from build123d import *

# Parameters (mm, degrees)
SKETCH1_W               = 85
SKETCH1_H               = 85
SKETCH1_W_2             = 20
SKETCH1_H_2             = 25
BOSS_EXTRUDE1_DEPTH     = 42
CUT_EXTRUDE1_DEPTH      = 108.686284851
CUT_EXTRUDE2_DEPTH      = 122.642881801
CUT_EXTRUDE3_START      = -85
CUT_EXTRUDE3_DEPTH      = 85
SKETCH6_W               = 67
SKETCH6_H               = 42
CUT_EXTRUDE4_DEPTH      = 35
FILLET1_R               = 3
FILLET2_R               = 3
CUT_EXTRUDE6_DEPTH      = 107.514112815
CUT_EXTRUDE6_DEPTH_BACK = 107.514112815
M5_TAPPED_HOLE2_D       = 4.2
M5_TAPPED_HOLE2_DEPTH   = 8
M5_TAPPED_HOLE2_TIP     = 1.2618073
SKETCH17_R              = 2.5
CUT_EXTRUDE7_DEPTH      = 107.922102397


# Read off the part's stored shape, not the designer's step: Cut-Extrude3
with BuildPart() as part:
    # Sketch1 → Boss-Extrude1 (new body)
    with BuildSketch(Plane(origin=(0, 0, 0), x_dir=(1, 0, 0), z_dir=(0, 1, 0))):
        with Locations((-20.937727355, 33.710174471)):
            Rectangle(SKETCH1_W, SKETCH1_H)
        with Locations((-53.437727355, -21.289825529)):
            Rectangle(SKETCH1_W_2, SKETCH1_H_2)
        with Locations((11.562272645, -21.289825529)):
            Rectangle(SKETCH1_W_2, SKETCH1_H_2)
    extrude(amount=BOSS_EXTRUDE1_DEPTH)

    # Sketch2 → Cut-Extrude1 (cut, through all)
    with BuildSketch(Plane(origin=(0, 42, 0), x_dir=(1, 0, 0), z_dir=(0, 1, 0))):
        with BuildLine():
            Line((-63.437727355, -23.334516424), (-63.437727355, -33.789825529))
            Line((-63.437727355, -33.789825529), (-43.437727355, -33.789825529))
            Line((-43.437727355, -33.789825529), (-43.437727355, -23.334516424))
            ThreePointArc((-43.437727355, -23.334516424), (-53.437727355, -33.334516424), (-63.437727355, -23.334516424))
        make_face()
        with BuildLine():
            Line((1.562272645, -23.334516424), (1.562272645, -33.789825529))
            Line((1.562272645, -33.789825529), (21.562272645, -33.789825529))
            Line((21.562272645, -33.789825529), (21.562272645, -23.334516424))
            ThreePointArc((21.562272645, -23.334516424), (11.562272645, -33.334516424), (1.562272645, -23.334516424))
        make_face()
    extrude(amount=-CUT_EXTRUDE1_DEPTH, mode=Mode.SUBTRACT)

    # Sketch3 → Cut-Extrude2 (cut, through all)
    with BuildSketch(Plane.ZY.offset(63.437727355)):
        Polygon((33.334516424, 2), (15.334516424, 2), (10.589618013, 0), (33.334516424, 0), align=None)
        Polygon((15.334516424, 40), (10.589618013, 42), (33.334516424, 42), (33.334516424, 40), align=None)
    extrude(amount=-CUT_EXTRUDE2_DEPTH, mode=Mode.SUBTRACT)

    # Cut-Extrude3 outline → Cut-Extrude3 (cut)
    with BuildSketch(Plane.ZY.offset(63.437727355).offset(CUT_EXTRUDE3_START)):
        with BuildLine():
            Line((33.334516424, 5.260289026), (33.334516424, 36.739710974))
            Line((33.334516424, 36.739710974), (5.643342669, 36.739710974))
            ThreePointArc((5.643342669, 36.739710974), (-13.23093958, 21), (5.643342669, 5.260289026))
            Line((5.643342669, 5.260289026), (33.334516424, 5.260289026))
        make_face()
    extrude(amount=CUT_EXTRUDE3_DEPTH, mode=Mode.SUBTRACT)

    # Sketch6 → Cut-Extrude4 (cut)
    with BuildSketch(Plane(origin=(0, 0, -76.210174471), x_dir=(-1, 0, 0), z_dir=(0, 0, -1))):
        with Locations((20.937727355, 21)):
            Rectangle(SKETCH6_W, SKETCH6_H)
    extrude(amount=-CUT_EXTRUDE4_DEPTH, mode=Mode.SUBTRACT)

    # Fillet1
    # the kernel refuses this fillet: 3 mm, written as the material it takes off along each edge
    with BuildSketch(Plane(origin=(-63.437727355, 42, -94.210174471), x_dir=(1, 0, 0), z_dir=(0, 0, 1)), Plane(origin=(-63.437727355, 0, 28.589618013), x_dir=(1, 0, 0), z_dir=(0, 0, -1)), Plane(origin=(21.562272645, 42, -94.210174471), x_dir=(0, -1, 0), z_dir=(0, 0, 1)), Plane(origin=(21.562272645, 0, 28.589618013), x_dir=(0, 1, 0), z_dir=(0, 0, -1))) as fillet1_piece_1:
        with BuildLine():
            CenterArc((FILLET1_R, -FILLET1_R), FILLET1_R, 90, 90)
            Line((0, -FILLET1_R), (-FILLET1_R * 0.02, -FILLET1_R))
            Line((-FILLET1_R * 0.02, -FILLET1_R), (-FILLET1_R * 0.02, FILLET1_R * 0.02))
            Line((-FILLET1_R * 0.02, FILLET1_R * 0.02), (FILLET1_R, FILLET1_R * 0.02))
            Line((FILLET1_R, FILLET1_R * 0.02), (FILLET1_R, 0))
        make_face()
    extrude(amount=122.799792484, mode=Mode.SUBTRACT)

    # Fillet2
    fillet2_edges = [part.edges().sort_by_distance(p)[0] for p in [
        (12.562272645, 21, -41.210174471),
        (-54.437727355, 21, -41.210174471),
    ]]
    fillet(fillet2_edges, radius=FILLET2_R)

    # Sketch9 → Cut-Extrude6 (cut, two sides: drawn at the far end of the back side and taken through both)
    with BuildSketch(Plane(origin=(0, 0, -41.210174471), x_dir=(-1, 0, 0), z_dir=(0, 0, -1)).offset(-CUT_EXTRUDE6_DEPTH_BACK)):
        with BuildLine():
            Line((35.10328306, 7.804043613), (6.77217165, 7.804043613))
            ThreePointArc((6.77217165, 7.804043613), (3.236637744, 9.268509707), (1.77217165, 12.804043613))
            Line((1.77217165, 12.804043613), (1.77217165, 29.195956387))
            ThreePointArc((1.77217165, 29.195956387), (3.236637744, 32.731490293), (6.77217165, 34.195956387))
            Line((6.77217165, 34.195956387), (35.10328306, 34.195956387))
            ThreePointArc((35.10328306, 34.195956387), (38.638816966, 32.731490293), (40.10328306, 29.195956387))
            Line((40.10328306, 29.195956387), (40.10328306, 12.804043613))
            ThreePointArc((40.10328306, 12.804043613), (38.638816966, 9.268509707), (35.10328306, 7.804043613))
        make_face()
    extrude(amount=CUT_EXTRUDE6_DEPTH + CUT_EXTRUDE6_DEPTH_BACK, mode=Mode.SUBTRACT)

    # M5 Tapped Hole2
    with Locations(Plane(origin=(16.562272645, 29.5, -76.210174471), x_dir=(-1, 0, 0), z_dir=(0, 0, -1))):
        with Locations((0, 0), (0, -17), (75, -17), (75, 0)):
            Hole(M5_TAPPED_HOLE2_D / 2, depth=M5_TAPPED_HOLE2_DEPTH)
            with Locations((0, 0, -(M5_TAPPED_HOLE2_DEPTH + M5_TAPPED_HOLE2_TIP / 2))):  # 118° drill point
                Cone(0, M5_TAPPED_HOLE2_D / 2, M5_TAPPED_HOLE2_TIP, mode=Mode.SUBTRACT)

    # Sketch17 → Cut-Extrude7 (cut, through all)
    with BuildSketch(Plane(origin=(0, 40, 0), x_dir=(1, 0, 0), z_dir=(0, 1, 0))):
        with Locations(Location((-53.437727355, -24.203700837, 0), (0, 0, 270))):
            Circle(SKETCH17_R)
        with Locations(Location((11.562272645, -24.203700837, 0), (0, 0, 270))):
            Circle(SKETCH17_R)
    extrude(amount=-CUT_EXTRUDE7_DEPTH, mode=Mode.SUBTRACT)


solid = part.part
Could you check a few things on this model? Use its own coordinates, in mm. A direction names the side the tool comes from. Coordinates: 2 decimals unless noted, no trailing zeros. Order: outer loops, then holes, each group sorted by start corner. A loop starts at its lowest first (then second) coordinate and runs counter-clockwise, first axis right, second up. Notation, with made-up numbers: (-31.75, -21.5) - (5.25, -21.5) arc R7 cw to (5.25, -13.5) - close; hole circle Ø6 at (-35.75, 75.5). An arc over 180 degrees is marked (long way). Answer in a Markdown table with one row per item. Add a question column.
(1) If we section it at B-B, the plane y = 21: Please give me the cut outline in (x, z), then the cut area to 3 significant figures.
(2) If we section it at C-C, the plane x = -5.5: Please give me the cut outline in (y, z).
(3) I need wall thicknesses on L1, parallel to X at y = 29.5, z = -70; L2, parallel to X at y = 34, z = -65; L3, parallel to Y at x = -23.5, z = 7. Which ranges of each line are inside material? Lowest first, please.
(4) If we mould it in two halves opening along Y, with no side actions, what happens to faces 1 (the face through (1.562, 3, 16)), 2 (the face through (-21, 42, -24)), 3 (the face through (-38.68, 9.31, -23.5))? For each: released by +Y, released by -Y, zero draft, split by the parting line, or undercut.
(5) Will these pins go through, and if not, where does the flat tip stop? pin 1 (1 mm diameter, centred on x = -27.5, y = 8.5, fed in from +Z); pin 2 (5.5 mm diameter, centred on x = -58.44, y = 12.5, fed in from +Z); pin 3 (2.5 mm diameter, centred on y = 1.5, z = 13.5, fed in from -X); pin 4 (5.5 mm diameter, centred on x = 7.5, z = 26.5, fed in from -Y).
(6) If we section it at A-A, the plane z = -37.5: Please give me the cut outline in (x, y).
(7) If we section it at D-D, the plane z = 7.5: Please give me the cut outline in (x, y), then the cut area to 3 significant figures.
(8) On a 3-axis mill with a long thin cutter (end or side, diameter ignored), from which of +Z, -Z, +X, -X, +Y, -Y can I reach the whole of each face in a straight line? I mean faces 4 (the face through (12.562, 21, -60)), 5 (the face through (-20, 36.74, 7)), 6 (the face through (-38.6, 32.77, -23.5)), 7 (the face through (-56.498, 11.696, -72.154)), 8 (the face through (-43.438, 3, 16)). Say none if no direction works.
Results are:
| question | item | result |
|---|---|---|
| 1 | outline | (-63.44, -76.21) - (-54.44, -76.21) - (-54.44, -44.21) arc R3 cw to (-51.44, -41.21) - (-40.1, -41.21) - (-40.1, -13.23) - (-63.44, -13.23) - close; (-1.77, -41.21) - (9.56, -41.21) arc R3 cw to (12.56, -44.21) - (12.56, -76.21) - (21.56, -76.21) - (21.56, -13.23) - (-1.77, -13.23) - close |
| 1 | area | 1,940 mm2 |
| 2 | outline | (0, -41.21) - (7.97, -41.21) - (7.97, -6.51) arc R16 cw to (5.26, 5.64) - (5.26, 8.79) - (0, 8.79) - close; (34.03, -41.21) - (42, -41.21) - (42, 8.79) - (36.74, 8.79) - (36.74, 5.64) arc R16 cw to (34.03, -6.51) - close |
| 3 | L1 | x = -63.44 to -60.54, -56.34 to -54.44, 12.56 to 14.46, 18.66 to 21.56 |
| 3 | L2 | x = -63.44 to -54.44, 12.56 to 21.56 |
| 3 | L3 | y = 0 to 5.26, 36.74 to 42 |
| 4 | face 1 | zero draft |
| 4 | face 2 | released by +Y |
| 4 | face 3 | undercut |
| 5 | pin 1 | passes through |
| 5 | pin 2 | stops at z = -8.61 |
| 5 | pin 3 | stops at x = -63.43 |
| 5 | pin 4 | stops at y = 2 |
| 6 | outline | (-63.44, 3) arc R3 ccw to (-60.44, 0) - (18.56, 0) arc R3 ccw to (21.56, 3) - (21.56, 39) arc R3 ccw to (18.56, 42) - (-60.44, 42) arc R3 ccw to (-63.44, 39) - close; hole (-40.1, 12.8) arc R5 ccw to (-35.1, 7.8) - (-6.77, 7.8) arc R5 ccw to (-1.77, 12.8) - (-1.77, 29.2) arc R5 ccw to (-6.77, 34.2) - (-35.1, 34.2) arc R5 ccw to (-40.1, 29.2) - close |
| 7 | outline | (-63.44, 3) arc R3 ccw to (-60.44, 0) - (18.56, 0) arc R3 ccw to (21.56, 3) - (21.56, 5.26) - (-63.44, 5.26) - close; (-63.44, 36.74) - (21.56, 36.74) - (21.56, 39) arc R3 ccw to (18.56, 42) - (-60.44, 42) arc R3 ccw to (-63.44, 39) - close |
| 7 | area | 887 mm2 |
| 8 | face 4 | -Z, +Y, -Y |
| 8 | face 5 | +Z, +X, -X |
| 8 | face 6 | +Z, -Z |
| 8 | face 7 | -Z |
| 8 | face 8 | +Z, +Y, -Y |
